Verification items for the finished model (mm, model axes). Round coordinates to 2 decimals unless told otherwise and drop trailing zeros. Order: outer loops, then holes, each group sorted by start corner. A loop starts at its lowest first (then second) coordinate and runs counter-clockwise, first axis right, second up. Notation, with made-up numbers: (42.25, -4.75) -> (79.25, -4.75) arc R31 cw to (79.25, 34.25) -> close; hole circle Ø2 at (28, 17.5). An arc over 180 degrees is marked (long way). Put each result on its own line as item: value.
```python
from build123d import *

# Parameters (mm, degrees)
SKETCH1_R               = 30.1625
SKETCH1_R_2             = 26.2509
BOSS_EXTRUDE1_DEPTH     = 747.903150098
CUT_EXTRUDE1_DEPTH      = 750.11859858
CUT_EXTRUDE1_DEPTH_BACK = 750.11859858
SKETCH2_W               = 57.15
SKETCH2_H               = 19.05


with BuildPart() as part:
    # Sketch1 → Boss-Extrude1 (new body)
    with BuildSketch(Plane.XY):
        with Locations(Location((0, 0, 0), (0, 0, 270))):
            Circle(SKETCH1_R)
        with Locations(Location((0, 0, 0), (0, 0, 270))):
            Circle(SKETCH1_R_2, mode=Mode.SUBTRACT)
    extrude(amount=BOSS_EXTRUDE1_DEPTH)

    # Sketch2 → Cut-Extrude1 (cut, two sides: drawn at the far end of the back side and taken through both)
    with BuildSketch(Plane(origin=(0, 0, 0), x_dir=(0, 0, -1), z_dir=(1, 0, 0)).offset(-CUT_EXTRUDE1_DEPTH_BACK)):
        Polygon((-732.028150098, -21.648424474), (-687.578150098, -21.648424474), (-687.578150098, -40.698424474), (-732.028150098, -40.698424474), (-757.696723695, -40.698424474), (-757.696723695, -21.648424474), align=None)
        with Locations((-493.303150098, -31.173424474)):
            Rectangle(SKETCH2_W, SKETCH2_H)
    extrude(amount=CUT_EXTRUDE1_DEPTH + CUT_EXTRUDE1_DEPTH_BACK, mode=Mode.SUBTRACT)


solid = part.part
```
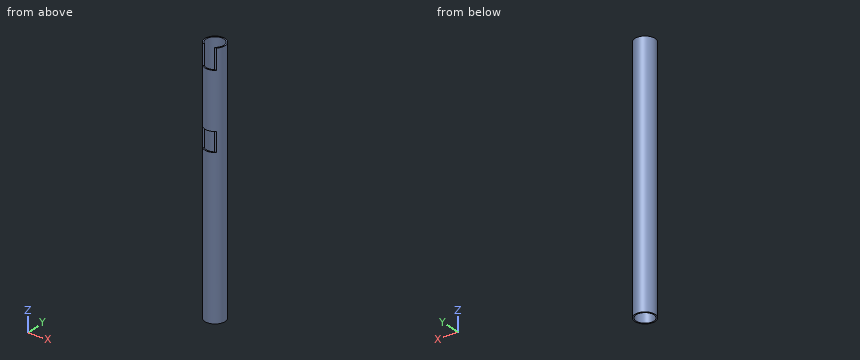
Item 1: Material ranges on line 1 along Y through (x, z) = (0, 563); line 2 along X through (y, z) = (2, 710), recorded low to high.
Geometry check:
line 1: -30.16 to -26.25, 26.25 to 30.16
line 2: -30.1 to -26.17, 26.17 to 30.1
Item 2: Sectioned sample at A-A, the plane x = 0. Record the boundary of the cut face in (y, z).
Geometry check:
outline: (-30.16, 0) -> (-26.25, 0) -> (-26.25, 464.73) -> (-30.16, 464.73) -> close; (-30.16, 521.88) -> (-26.25, 521.88) -> (-26.25, 687.58) -> (-30.16, 687.58) -> close; (26.25, 0) -> (30.16, 0) -> (30.16, 747.9) -> (26.25, 747.9) -> close
Item 3: Depth check by flat-ended pin: pin 1 Ø7 at (x, y) = (0.5, -26) entering from +Z; pin 2 Ø6 at (y, z) = (-19, 659) entering from +X; pin 3 Ø3 at (x, z) = (-18, 506) entering from -Y; pin 4 Ø7 at (x, y) = (2, -25.5) entering from -Z. Enter the tip coordinate at first touch or a pass-through.
Geometry check:
pin 1: z = 687.58
pin 2: x = 25.57
pin 3: y = -21.65
pin 4: z = 0
Item 4: Sectioned sample at C-C, the plane z = 191.5. Record the boundary of the cut face in (x, y) (1 decimal), then the cut area to 3 significant figures.
Geometry check:
outline: circle Ø60.3 at (0, 0); hole circle Ø52.5 at (0, 0)
area: 693 mm2
Item 5: Sectioned sample at B-B, the plane y = 0. Record the boundary of the cut face in (x, z), then the cut area to 3 significant figures.
Geometry check:
outline: (-30.16, 0) -> (-26.25, 0) -> (-26.25, 747.9) -> (-30.16, 747.9) -> close; (26.25, 0) -> (30.16, 0) -> (30.16, 747.9) -> (26.25, 747.9) -> close
area: 5,850 mm2
